Check sheet for the modelled part. Datum: model origin and axes. Units: mm. Round coordinates to 2 decimals unless told otherwise and drop trailing zeros. Write each loop counter-clockwise with the first axis right and the second up, starting at its lowest first coordinate (ties: lowest second). Pieces come first, ordered by that corner, then holes. Notation, with made-up numbers: (38.5, -22.5) -> (84.5, -22.5) arc R22 cw to (84.5, 16.5) -> close; hole circle Ø11 at (-10, -29). An arc over 180 degrees is marked (long way). Put each result on its own line as item: value. Start each with the question number.
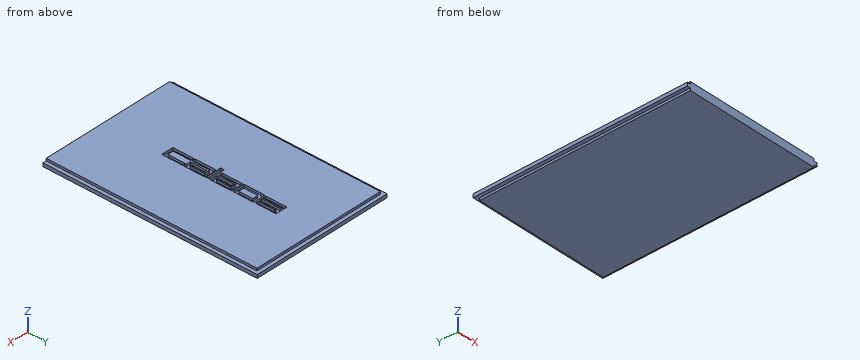
from build123d import *

# Parameters (mm, degrees)
SKETCH_W      = 61.5
SKETCH_H      = 93
PAD_DEPTH     = 1.5
SKETCH001_W   = 58.5
SKETCH001_H   = 91.5
PAD001_DEPTH  = 1
SKETCH002_W   = 58.5
SKETCH002_H   = 91.5
PAD002_DEPTH  = 1
SKETCH003_W   = 5.409756
SKETCH003_H   = 9.051441
SKETCH003_W_2 = 2.375015
SKETCH003_H_2 = 6.06948
SKETCH003_W_3 = 1.477786
SKETCH003_H_3 = 9.209776
POCKET_DEPTH  = 1


with BuildPart() as part:
    # Sketch → Pad (new body)
    with BuildSketch(Plane.XY):
        Rectangle(SKETCH_W, SKETCH_H)
    extrude(amount=PAD_DEPTH)

    # Sketch001 → Pad001 (new body)
    with BuildSketch(Plane.XY.offset(1.5)):
        with Locations((0, -0.75)):
            Rectangle(SKETCH001_W, SKETCH001_H)
    extrude(amount=PAD001_DEPTH)

    # Sketch002 → Pad002 (new body)
    with BuildSketch(Plane(origin=(0, 0, 0), x_dir=(1, 0, 0), z_dir=(0, 0, -1))):
        with Locations((0, 0.75)):
            Rectangle(SKETCH002_W, SKETCH002_H)
    extrude(amount=PAD002_DEPTH)

    # Sketch003 → Pocket (cut)
    with BuildSketch(Plane.XY.offset(2.5)):
        Polygon((-2.621542, -11.556755), (-1.143755, -11.556755), (-1.143755, -19.262356), (1.310425, -19.262356), (1.310425, -11.530366), (2.629878, -11.530366), (2.629878, -20.713753), (-2.621542, -20.713753), align=None)
        Polygon((-2.647752, -11.18105), (-1.143755, -11.18105), (-1.143755, -3.376151), (1.257648, -3.376151), (1.257648, -9.735911), (0.756256, -9.735911), (0.756256, -3.930321), (-0.45764, -3.930321), (-0.45764, -11.16092), (2.709045, -11.16092), (2.709045, -1.892107), (-2.647752, -1.892107), align=None)
        Polygon((-4.495397, -0.064355), (2.471311, -0.064355), (2.550478, -1.647698), (-4.495397, -1.647698), align=None)
        Polygon((-2.675537, 0.499041), (-1.196766, 0.499041), (-1.196766, 8.063471), (1.257415, 8.063471), (1.257415, 1.835656), (0.756023, 1.835656), (0.756023, 7.641245), (-0.642597, 7.641245), (-0.642597, 0.489815), (2.682424, 0.489815), (2.682424, 9.576872), (-2.675537, 9.576872), align=None)
        with Locations((-0.076145, 14.5865)):
            Rectangle(SKETCH003_W, SKETCH003_H)
        with Locations((0.095295, 14.504397)):
            Rectangle(SKETCH003_W_2, SKETCH003_H_2, mode=Mode.SUBTRACT)
        with Locations((-1.857495, 24.255149)):
            Rectangle(SKETCH003_W_3, SKETCH003_H_3)
        Polygon((-0.59082, 19.571095), (-0.59082, 28.833649), (2.549475, 28.833649), (2.549475, 19.729427), (1.203635, 19.729427), (1.203635, 27.250305), (0.728631, 27.250305), (0.728631, 19.729427), align=None)
    extrude(amount=-POCKET_DEPTH, mode=Mode.SUBTRACT)


solid = part.part
1. Material ranges on L1, parallel to X at y = -5.5, z = 2; L2, parallel to X at y = -12, z = 1.6; L3, parallel to Y at x = 9, z = 2.3, recorded low to high. Write a range as [from, to].
2. Gauge pin test, flat ends, axial feed: P1, Ø0.5, axis at y = 24.5, z = 2, coming from the -X side; P2, Ø0.5, axis at y = -14, z = 2, coming from the +X side; P3, Ø0.5, axis at x = -2, z = 2, coming from the +Y side. Record the tip position at first contact, or that the pin passes through.
3. Section check B-B, the plane y = -23.5. Enter the section's corners in (x, z).
4. Section check A-A, the plane y = 6.5. Enter the section's corners in (x, z).
Reply:
1. L1: x = [-29.25, -2.65], [-1.14, -0.46], [0.76, 1.26], [2.71, 29.25]
1. L2: x = [-29.25, -2.62], [-1.14, 1.31], [2.63, 29.25]
1. L3: y = [-46.5, 45]
2. P1: stops at x = -29.25
2. P2: stops at x = 29.25
2. P3: stops at y = 45
3. outline: (-30.75, 0) -> (-29.25, 0) -> (-29.25, -1) -> (29.25, -1) -> (29.25, 0) -> (30.75, 0) -> (30.75, 1.5) -> (29.25, 1.5) -> (29.25, 2.5) -> (-29.25, 2.5) -> (-29.25, 1.5) -> (-30.75, 1.5) -> close
4. outline: (-30.75, 0) -> (-29.25, 0) -> (-29.25, -1) -> (29.25, -1) -> (29.25, 0) -> (30.75, 0) -> (30.75, 1.5) -> (29.25, 1.5) -> (29.25, 2.5) -> (2.68, 2.5) -> (2.68, 1.5) -> (1.26, 1.5) -> (1.26, 2.5) -> (0.76, 2.5) -> (0.76, 1.5) -> (-0.64, 1.5) -> (-0.64, 2.5) -> (-1.2, 2.5) -> (-1.2, 1.5) -> (-2.68, 1.5) -> (-2.68, 2.5) -> (-29.25, 2.5) -> (-29.25, 1.5) -> (-30.75, 1.5) -> close
